Input: dimensioned drawing with shaded views. Units: mm. Origin: part minimum x, y, z. A direction names the side the tool comes from. Give positions to 0.01 mm unless a question says otherwise; leave off trailing zeros. Write each loop counter-clockwise with the first axis right and the second up, starting at its lowest first coordinate (ties: lowest second). Pieces come first, ordered by that corner, then holes. Notation, with made-up numbers: (87.25, 51.5) -> (94.25, 51.5) arc R30 cw to (94.25, 87.5) -> close; hole circle Ø7 at (14, 69). An arc over 180 degrees is marked (long way). Return JSON: item names as keys, results as strings. Group by question number.
Item 1: Section B-B, the plane x = 6. Return loops of the section in (y, z).
Item 2: Mould query, pull axis Z, two halves, no side actions, for the marked faces 3, 4 and 5. Classes: released by +Z, released by -Z, zero draft, split by the parting line, or undercut.
Item 3: Set-up query: the marked faces 1 and 2. Return all of +Z, -Z, +X, -X, +Y, -Y with unobstructed straight access to the full face (end or side cutting, diameter ignored); none if empty.
Item 4: Line query: line 1 (X direction, y = 1.8, z = 20); line 2 (Z direction, x = 13, y = 2.3) (1 decimal); line 3 (Z direction, x = 20.5, y = 5.5) (1 decimal). Output: solid intervals per line, ascending. Write a range as [from, to].
Item 5: Section A-A, the plane y = 5. Return loops of the section in (x, z).
Item 6: Section D-D, the plane z = 29. Return loops of the section in (x, y).
Item 7: Pin query (flat end, axial travel): P1, Ø7, axis at x = 13, z = 32.12, coming from the +Y side; P2, Ø3, axis at x = 26.5, z = 20, coming from the -Y side; P3, Ø2.5, axis at x = 27, z = 32.12, coming from the -Y side; P4, Ø10, axis at y = 11.5, z = 21.5, coming from the +X side. Return the tip coordinate at first contact, or that it passes through.
Item 8: Section C-C, the plane y = 1.25. Count the separate pieces of the cut face and the enclosed holes in it, then the cut area to 3 significant figures.
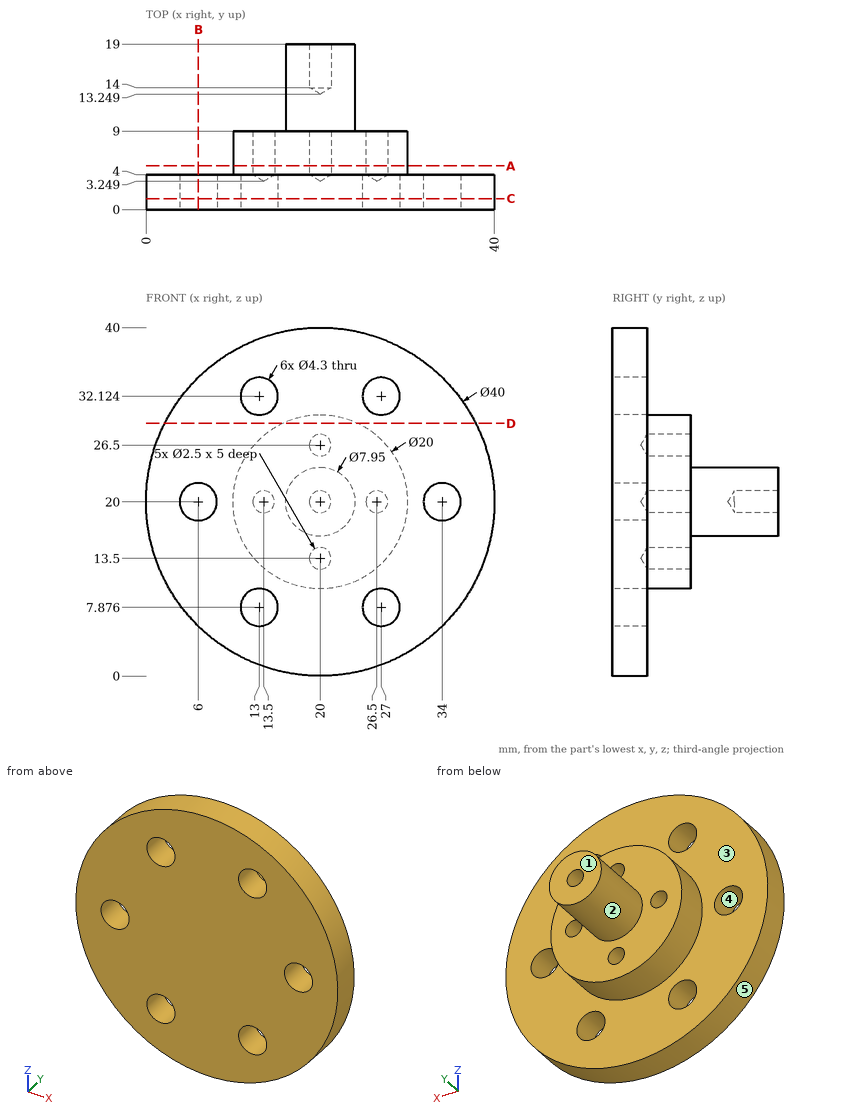
Answer below:
{
 "1": {"outline": "(0, 5.72) -> (4, 5.72) -> (4, 17.85) -> (0, 17.85) -> close; (0, 22.15) -> (4, 22.15) -> (4, 34.28) -> (0, 34.28) -> close"},
 "2": {"face 3": "zero draft", "face 4": "undercut", "face 5": "split by the parting line"},
 "3": {"face 1": "+Z, -Z, +X, -X, +Y", "face 2": "+Y"},
 "4": {"line 1": "x = [0, 3.85], [8.15, 31.85], [36.15, 40]", "line 2": "z = [1.3, 5.7], [10, 30], [34.3, 38.7]", "line 3": "z = [10, 12.4], [14.6, 25.4], [27.6, 30]"},
 "5": {"outline": "circle Ø20 at (20, 20); hole circle Ø2.5 at (13.5, 20); hole circle Ø2.5 at (20, 13.5); hole circle Ø2.5 at (20, 26.5); hole circle Ø2.5 at (26.5, 20)"},
 "6": {"outline": "(2.14, 0) -> (37.86, 0) -> (37.86, 4) -> (24.36, 4) -> (24.36, 9) -> (15.64, 9) -> (15.64, 4) -> (2.14, 4) -> close"},
 "7": {"P1": "stops at y = 4", "P2": "stops at y = 0", "P3": "passes through", "P4": "stops at x = 30"},
 "8": {"separate pieces": "1", "enclosed holes": "6", "area": "1,170 mm2"}
}
